Could you check a few things on this drawing? It's one solid part, dimensions in mm from its lowest x, y, z. Round coordinates to 2 decimals unless told otherwise and drop trailing zeros. Write each loop counter-clockwise with the first axis right and the second up, starting at its lowest first coordinate (ties: lowest second). Pieces come first, ordered by that corner, then holes. Notation, with made-up numbers: (47.5, -21) - (106.5, -21) arc R20 cw to (106.5, -9) - close; hole circle Ø8 at (81, 67.25). An arc over 180 degrees is marked (long way). Use one line per item in the form item = value. Start each with the question number.
1. Will this pin go through, and if not, where does the flat tip stop? pin 1 (2.5 mm diameter, centred on x = 40, y = 5, fed in from -Z).
2. I want a section at B-B, the plane x = 10. List the corners of the cut face in (y, z) for me.
3. I want a section at D-D, the plane x = 26. List the corners of the cut face in (y, z) for me.
4. I want a section at C-C, the plane y = 5.5. List the corners of the cut face in (x, z) for me (1 decimal), plus the area to 3 significant figures.
5. I want a section at A-A, the plane z = 1.75. State how many separate pieces and enclosed holes the cut face has, plus the area to 3 significant figures.
6. If I drill on line 1 along X through (y, z) = (3.5, 4.5); line 2 along Y through (x, z) = (10, 1.8); line 3 along X through (y, z) = (3.25, 1.95), over which ranges is the centre line in solid material (lowest first)?
7. We'd pull the mould along X, two halves only. Please class the marked faces 1, 2 and 3: +X half, -X half, draft (parallel to the pull), parting line (faces both ways), or undercut.
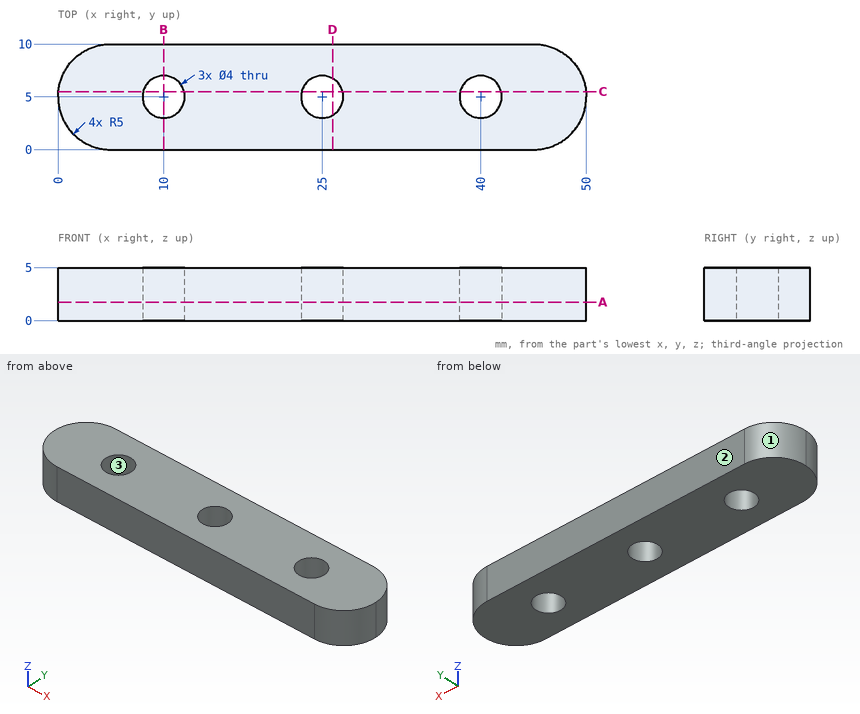
Model answer:
q1.pin_1 = through
q2.outline = (0, 0) - (3, 0) - (3, 5) - (0, 5) - close; (7, 0) - (10, 0) - (10, 5) - (7, 5) - close
q3.outline = (0, 0) - (3.27, 0) - (3.27, 5) - (0, 5) - close; (6.73, 0) - (10, 0) - (10, 5) - (6.73, 5) - close
q4.outline = (0, 0) - (8.1, 0) - (8.1, 5) - (0, 5) - close; (11.9, 0) - (23.1, 0) - (23.1, 5) - (11.9, 5) - close; (26.9, 0) - (38.1, 0) - (38.1, 5) - (26.9, 5) - close; (41.9, 0) - (50, 0) - (50, 5) - (41.9, 5) - close
q4.area = 192 mm2
q5.separate_pieces = 1
q5.enclosed_holes = 3
q5.area = 441 mm2
q6.line_1 = 0.23 to 8.68, 11.32 to 23.68, 26.32 to 38.68, 41.32 to 49.77
q6.line_2 = 0 to 3, 7 to 10
q6.line_3 = 0.32 to 9.03, 10.97 to 24.03, 25.97 to 39.03, 40.97 to 49.68
q7.face_1 = -X half
q7.face_2 = draft
q7.face_3 = undercut
